```python
from build123d import *

# Parameters (mm, degrees)
F0_W     = 558.8
F0_H     = 627.0625
F0_W_2   = 6.35
F0_H_2   = 52.3875
F0_W_3   = 6.3499988437
F0_H_3   = 52.3875042677
F0_W_4   = 6.3500062943
F0_W_5   = 6.3499960899
F0_W_6   = 6.349999775
F0_W_7   = 6.3499979123
F1_DEPTH = 28.575
F2_W     = 546.1
F2_H     = 496.8875
F2_W_2   = 527.05
F2_H_2   = 477.8375
F2_W_3   = 520.7
F2_H_3   = 471.4875
F3_DEPTH = 11.1125
F4_DEPTH = 7.9375
F5_W     = 539.75
F5_H     = 490.5375
F5_W_2   = 533.4
F5_H_2   = 484.1875
F6_DEPTH = 17.4625
F7_R     = 1.5875
F8_DEPTH = 762


with BuildPart() as f1:
    # F0 (on Front) → F1 (new body)
    with BuildSketch(Plane.XZ):
        Rectangle(F0_W, F0_H)
        Polygon((-273.05, 254.79375), (-273.05, 307.18125), (-231.775, 307.18125), (-225.425, 307.18125), (-174.625, 307.18125), (-168.275, 307.18125), (-117.475, 307.18125), (-111.125, 307.18125), (-60.325, 307.18125), (-53.975, 307.18125), (-3.175, 307.18125), (3.175, 307.18125), (53.975, 307.18125), (60.325, 307.18125), (111.125, 307.18125), (117.475, 307.18125), (168.275, 307.18125), (174.625, 307.18125), (225.425, 307.18125), (231.775, 307.18125), (273.05, 307.18125), (273.05, 254.79375), (273.05, 248.44375), (273.05, -248.44375), (273.05, -254.7937457323), (273.05, -307.18125), (231.7750166416, -307.18125), (225.4250103474, -307.18125), (174.6250103474, -307.18125), (168.2750040531, -307.18125), (117.4750040531, -307.18125), (111.1249977589, -307.18125), (60.3249977589, -307.18125), (53.9749998465, -307.18125), (3.1749998465, -307.18125), (-3.1749999285, -307.18125), (-53.9749999285, -307.18125), (-60.3249987721, -307.18125), (-111.1249987721, -307.18125), (-117.4749976158, -307.18125), (-168.2749976158, -307.18125), (-174.6250039101, -307.18125), (-225.4250039101, -307.18125), (-231.775, -307.18125), (-273.05, -307.18125), (-273.05, -254.7937457323), (-273.05, -248.44375), (-273.05, 248.44375), align=None, mode=Mode.SUBTRACT)
        with Locations((-228.6, 280.9875)):
            Rectangle(F0_W_2, F0_H_2)
        with Locations((-171.45, 280.9875)):
            Rectangle(F0_W_2, F0_H_2)
        with Locations((-114.3, 280.9875)):
            Rectangle(F0_W_2, F0_H_2)
        with Locations((-57.15, 280.9875)):
            Rectangle(F0_W_2, F0_H_2)
        with Locations((0, 280.9875)):
            Rectangle(F0_W_2, F0_H_2)
        with Locations((57.15, 280.9875)):
            Rectangle(F0_W_2, F0_H_2)
        Polygon((-231.775, 254.79375), (-273.05, 254.79375), (-273.05, 248.44375), (273.05, 248.44375), (273.05, 254.79375), (231.775, 254.79375), (225.425, 254.79375), (174.625, 254.79375), (168.275, 254.79375), (117.475, 254.79375), (111.125, 254.79375), (60.325, 254.79375), (53.975, 254.79375), (3.175, 254.79375), (-3.175, 254.79375), (-53.975, 254.79375), (-60.325, 254.79375), (-111.125, 254.79375), (-117.475, 254.79375), (-168.275, 254.79375), (-174.625, 254.79375), (-225.425, 254.79375), align=None)
        with Locations((114.3, 280.9875)):
            Rectangle(F0_W_2, F0_H_2)
        with Locations((171.45, 280.9875)):
            Rectangle(F0_W_2, F0_H_2)
        Polygon((273.05, -248.44375), (-273.05, -248.44375), (-273.05, -254.7937457323), (-231.775, -254.7937457323), (-225.4250039101, -254.7937457323), (-174.6250039101, -254.7937457323), (-168.2749976158, -254.7937457323), (-117.4749976158, -254.7937457323), (-111.1249987721, -254.7937457323), (-60.3249987721, -254.7937457323), (-53.9749999285, -254.7937457323), (-3.1749999285, -254.7937457323), (3.1749998465, -254.7937457323), (53.9749998465, -254.7937457323), (60.3249977589, -254.7937457323), (111.1249977589, -254.7937457323), (117.4750040531, -254.7937457323), (168.2750040531, -254.7937457323), (174.6250103474, -254.7937457323), (225.4250103474, -254.7937457323), (231.7750166416, -254.7937457323), (273.05, -254.7937457323), align=None)
        with Locations((-114.299998194, -280.9874978662)):
            Rectangle(F0_W_3, F0_H_3)
        with Locations((-171.4500007629, -280.9874978662)):
            Rectangle(F0_W_4, F0_H_3)
        with Locations((-228.600001955, -280.9874978662)):
            Rectangle(F0_W_5, F0_H_3)
        with Locations((-57.1499993503, -280.9874978662)):
            Rectangle(F0_W_3, F0_H_3)
        with Locations((-4.1e-08, -280.9874978662)):
            Rectangle(F0_W_6, F0_H_3)
        with Locations((57.1499988027, -280.9874978662)):
            Rectangle(F0_W_7, F0_H_3)
        with Locations((114.300000906, -280.9874978662)):
            Rectangle(F0_W_4, F0_H_3)
        with Locations((171.4500072002, -280.9874978662)):
            Rectangle(F0_W_4, F0_H_3)
        with Locations((228.6000134945, -280.9874978662)):
            Rectangle(F0_W_4, F0_H_3)
        with Locations((228.6, 280.9875)):
            Rectangle(F0_W_2, F0_H_2)
    extrude(amount=F1_DEPTH)

    # F2 (on face) → F3 (join)
    with BuildSketch(Plane(origin=(0, 0, 0), x_dir=(-1, 0, 0), z_dir=(0, 1, 0))):
        Rectangle(F2_W, F2_H)
        Rectangle(F2_W_2, F2_H_2, mode=Mode.SUBTRACT)
        Rectangle(F2_W_2, F2_H_2)
        Rectangle(F2_W_3, F2_H_3, mode=Mode.SUBTRACT)
    extrude(amount=-F3_DEPTH)

    # F2 (on face) → F4 (cut)
    with BuildSketch(Plane(origin=(0, 0, 0), x_dir=(-1, 0, 0), z_dir=(0, 1, 0))):
        Rectangle(F2_W, F2_H)
        Rectangle(F2_W_2, F2_H_2, mode=Mode.SUBTRACT)
    extrude(amount=-F4_DEPTH, mode=Mode.SUBTRACT)

    # F5 (on face) → F6 (join)
    with BuildSketch(Plane.XZ.offset(11.1125)):
        Rectangle(F5_W, F5_H)
        Rectangle(F5_W_2, F5_H_2, mode=Mode.SUBTRACT)
    extrude(amount=F6_DEPTH)

    # F7 (on face) → F8 (cut, symmetric)
    with BuildSketch(Plane(origin=(266.7, 0, 0), x_dir=(0, -1, 0), z_dir=(-1, 0, 0))):
        with Locations((23.01875, 191.29375)):
            Circle(F7_R)
        with Locations((23.01875, 68.10375)):
            Circle(F7_R)
        with Locations((23.01875, -191.29375)):
            Circle(F7_R)
        with Locations((23.01875, -68.10375)):
            Circle(F7_R)
    extrude(amount=F8_DEPTH, both=True, mode=Mode.SUBTRACT)


solid = f1.part
```
The listing builds one solid part. Answer for the finished solid, in the listing's coordinates (mm). A direction names the side the tool comes from. Give positions to 0.01 mm unless a question says otherwise; leave off trailing zeros. Answer as a JSON object with one key per item and string values. Group by question number.
Item 1: Determine the mould class of faces 3 (the flat face through (1, 0, -254)), 4 (the flat face through (60.325, -14, -281)) for opening direction Z: pulls with the +Z half, pulls with the -Z half, needs draft (parallel to the pull), parting line crosses it, or undercut.
Item 2: The part is cut by section A-A on y = -16.25. Give the number of separate pieces and of enclosed holes in the cut face, and give its area (3 significant figures).
Item 3: Consider L1, parallel to Z at x = 4, y = -24; L2, parallel to X at y = -6.5, z = 123 (3 decimals); L3, parallel to Z at x = 183, y = -6.5. Determine where each line is inside the solid, lowest interval first. Write a range as from..to.
Item 4: A tool of negligible diameter and unlimited length cuts with its end or side. For faces 1 (the flat face through (-4, -20, -242.094)), 2 (the flat face through (-86, -14, 307.181)), from which of +Z, -Z, +X, -X, +Y, -Y can it reach the whole face along a straight path? Write none if from no direction.
Result set:
{
 "1": {"face 3": "needs draft", "face 4": "undercut"},
 "2": {"separate pieces": "2", "enclosed holes": "22", "area": "34,300 mm²"},
 "3": {"L1": "-313.53..-307.18, -254.79..-248.44, -245.27..-242.09, 242.09..245.27, 248.44..254.79, 307.18..313.53", "L2": "-279.4..-273.05, -263.525..-260.35, 260.35..263.525, 273.05..279.4", "L3": "-313.53..-307.18, -254.79..-248.44, -238.92..-235.74, 235.74..238.92, 248.44..254.79, 307.18..313.53"},
 "4": {"face 1": "-Y", "face 2": "+Y, -Y"}
}
